For this review, take the finished solid that the model builds, in its own axes (mm). A direction names the side the tool comes from. Give positions to 0.01 mm unless a question says otherwise; leave off trailing zeros. Write each loop counter-clockwise with the first axis right and the second up, starting at its lowest first coordinate (ties: lowest second). Pieces come first, ordered by that corner, then holes.
from build123d import *

# Parameters (mm, degrees)
SKETCH1_R           = 4.25
BOSS_EXTRUDE1_DEPTH = 27
SKETCH2_R           = 5.25
BOSS_EXTRUDE2_DEPTH = 5
SKETCH7_R           = 1.75
CUT_EXTRUDE4_DEPTH  = 33
CUT_EXTRUDE6_DEPTH  = 4


with BuildPart() as part:
    # Sketch1 → Boss-Extrude1 (new body)
    with BuildSketch(Plane.XY):
        Circle(SKETCH1_R)
    extrude(amount=BOSS_EXTRUDE1_DEPTH)

    # Sketch2 → Boss-Extrude2 (add)
    with BuildSketch(Plane.XY.offset(27)):
        Circle(SKETCH2_R)
    extrude(amount=BOSS_EXTRUDE2_DEPTH)

    # Sketch7 → Cut-Extrude4 (cut, through all)
    with BuildSketch(Plane.XY.offset(32)):
        Circle(SKETCH7_R)
    extrude(amount=-CUT_EXTRUDE4_DEPTH, mode=Mode.SUBTRACT)

    # Sketch9 → Cut-Extrude6 (cut)
    with BuildSketch(Plane.XY.offset(32)):
        Polygon((0, 3.464101615), (-3, 1.732050808), (-3, -1.732050808), (0, -3.464101615), (3, -1.732050808), (3, 1.732050808), align=None)
    extrude(amount=-CUT_EXTRUDE6_DEPTH, mode=Mode.SUBTRACT)


solid = part.part
(1) We need section A-A (y = 0). Write out the cut boundary in (x, z).
(2) We need section D-D (y = 3). Write out the cut boundary in (x, z).
(3) The part is to be moulded in two halves that separate along Y. For faces 3 (the flat face through (2, -4, 27)), 4 (the cylindrical face through (2.285, 3.584, 13.311)), 5 (the flat face through (1.5, -2.6, 30)), say which applies: +Y half, -Y half, draft (parallel to the pull), parting line (faces both ways), or undercut.
(4) We need section C-C (z = 21.5). Write out the cut boundary in (x, y), and give its area (3 significant figures).
(5) Tool access review of faces 1 (the flat face through (-1.5, 2.6, 30)), 2 (the flat face through (2, 0, 0)): name each direction out of +Z, -Z, +X, -X, +Y, -Y from which nothing blocks a thin tool from reaching the whole face with its end or side.
(6) We need section B-B (x = 1). Write out the cut boundary in (y, z), and give its area (3 significant figures).
(7) Clearance check with flat-ended pins moving along their axes: pin 1 Ø4 at (x, z) = (-2.5, 15) entering from -Y; pin 2 Ø3 at (x, z) = (-2.5, 12.5) entering from +Y; pin 3 Ø3 at (y, z) = (-1, 15) entering from +X. State where each tip first meets the part, or that it passes through.
(8) For L1, parallel to Y at x = 0, z = 9; L2, parallel to Z at x = 0, y = -4.5; L3, parallel to Y at x = -1.25, z = 20, list the stretches that pass through material, from the lowest coordinate up.
The answers:
1. outline: (-5.25, 27) - (-4.25, 27) - (-4.25, 0) - (-1.75, 0) - (-1.75, 28) - (-3, 28) - (-3, 32) - (-5.25, 32) - close; (1.75, 0) - (4.25, 0) - (4.25, 27) - (5.25, 27) - (5.25, 32) - (3, 32) - (3, 28) - (1.75, 28) - close
2. outline: (-4.31, 27) - (-3.01, 27) - (-3.01, 0) - (3.01, 0) - (3.01, 27) - (4.31, 27) - (4.31, 32) - (0.8, 32) - (0.8, 28) - (-0.8, 28) - (-0.8, 32) - (-4.31, 32) - close
3. face 3: draft
3. face 4: parting line
3. face 5: undercut
4. outline: circle Ø8.5 at (0, 0); hole circle Ø3.5 at (0, 0)
4. area: 47.1 mm2
5. face 1: +Z
5. face 2: -Z, +X, -X, +Y, -Y
6. outline: (-5.15, 27) - (-4.13, 27) - (-4.13, 0) - (-1.44, 0) - (-1.44, 28) - (-2.89, 28) - (-2.89, 32) - (-5.15, 32) - close; (1.44, 0) - (4.13, 0) - (4.13, 27) - (5.15, 27) - (5.15, 32) - (2.89, 32) - (2.89, 28) - (1.44, 28) - close
6. area: 171 mm2
7. pin 1: stops at y = -4.22
7. pin 2: stops at y = 4.13
7. pin 3: stops at x = 4.25
8. L1: y = -4.25 to -1.75, 1.75 to 4.25
8. L2: z = 27 to 32
8. L3: y = -4.06 to -1.22, 1.22 to 4.06
